from build123d import *

# Parameters (mm, degrees)
F1_DEPTH     = 19.05
F2_T1_DEPTH  = 28.2300180496
F2_T3_DEPTH  = 25.482580603
F2_T5_DEPTH  = 25.9366089247
F2_T7_DEPTH  = 47.5485210799
F2_T9_DEPTH  = 32.7314977927
F2_T11_DEPTH = 59.1455336843
F2_T13_DEPTH = 52.8213628452
F2_T15_DEPTH = 21.9875710363
F2_T17_DEPTH = 46.4468482438
F2_T19_DEPTH = 29.758572197
F3_R         = 5.08
F5_W         = 6.35
F5_H         = 12.7
F6_DEPTH     = 303.0582275594


# Not quite as in the source:
# - a fillet or chamfer that OpenCascade refuses, or shapes differently, is made with other operations: its cross-section is extruded or revolved along the edge and cut away or added


with BuildPart() as f1:
    # F0 (on Front) → F1 (new body)
    with BuildSketch(Plane.XZ):
        Polygon((-45.0859302655, 0.4672128707), (-34.340060316, 0.4672128707), (-31.5367905423, 4.9057230353), (-31.5367905423, 9.1106286272), (-31.5367905423, 12.6147158444), (-29.4343372807, 13.7827442959), (-19.1556811333, 15.8851970918), (-16.2193404098, 14.3601642462), (-11.9138995651, 12.6147158444), (-11.9138995651, 9.1106286272), (-11.9138995651, 7.4753854424), (-9.811447002, 1.5152803213), (-6.0737542808, 0), (0, 0), (0, 2.3983575983), (1.1680293828, 5.2794977153), (1.1680293828, 9.1106286272), (1.1680293828, 12.6147158444), (0, 17.2868324444), (-1.4916199837, 18.4976548306), (3.0368734151, 29.6679423191), (4.9057211727, 31.0695767403), (6.0737496242, 31.770395115), (8.4476916948, 31.5367886797), (9.3986034807, 33.8823718767), (12.8483185545, 32.4838392109), (15.1843773201, 31.5367886797), (18.6884636059, 40.1802044362), (14.483560808, 40.1802044362), (14.483560808, 42.2826576978), (12.8483185545, 42.7498687059), (12.1475020424, 44.1515035927), (8.1762028858, 44.1515035927), (5.3729321808, 44.1515035927), (1.1680293828, 44.1515035927), (1.1680293828, 42.2826576978), (-1.4016367495, 40.4138118029), (-3.9712996222, 38.3113585413), (-14.7171695717, 38.3113585413), (-22.192556411, 38.3113585413), (-28.7335207686, 38.3113585413), (-38.0777539685, 35.5080878362), (-43.684293516, 32.4712125584), (-49.0572275594, 27.7990954928), (-49.0572275594, 14.9507736787), (-49.0572275594, 9.1106286272), align=None)
    extrude(amount=F1_DEPTH)

    # F2: fillet of radius 12.5094889948 on 10 edges, made by hand

    # F2_s2 → F2_t1 (cut)
    with BuildSketch(Plane.XZ.offset(-4.5900090248)):
        with BuildLine():
            ThreePointArc((-30.4920932473, 37.7837866574), (-28.7140598467, 38.1787628389), (-26.8975171587, 38.3113585413))
            Line((-26.8975171587, 38.3113585413), (-28.7335207686, 38.3113585413))
            Line((-28.7335207686, 38.3113585413), (-30.4920932473, 37.7837866574))
        make_face()
    extrude(amount=F2_T1_DEPTH, mode=Mode.SUBTRACT)

    # F2_s4 → F2_t3 (cut)
    with BuildSketch(Plane.XZ.offset(-3.2162903015)):
        with BuildLine():
            ThreePointArc((-39.2089772844, 34.8953419361), (-38.0524286269, 35.4471609705), (-36.8454950389, 35.8777656133))
            Line((-36.8454950389, 35.8777656133), (-38.0777539685, 35.5080878362))
            Line((-38.0777539685, 35.5080878362), (-39.2089772844, 34.8953419361))
        make_face()
    extrude(amount=F2_T3_DEPTH, mode=Mode.SUBTRACT)

    # F2_s6 → F2_t5 (cut)
    with BuildSketch(Plane.XZ.offset(-3.4433044624)):
        with BuildLine():
            ThreePointArc((-42.4732255071, 33.1272076629), (-43.6412308258, 32.4090824128), (-44.7236280922, 31.5674432638))
            Line((-44.7236280922, 31.5674432638), (-43.684293516, 32.4712125584))
            Line((-43.684293516, 32.4712125584), (-42.4732255071, 33.1272076629))
        make_face()
    extrude(amount=F2_T5_DEPTH, mode=Mode.SUBTRACT)

    # F2_s8 → F2_t7 (cut)
    with BuildSketch(Plane.XZ.offset(-14.2492605399)):
        with BuildLine():
            ThreePointArc((-49.0572275594, 22.0993912768), (-47.9313005389, 27.2860888474), (-44.7561994839, 31.5391203114))
            Line((-44.7561994839, 31.5391203114), (-49.0572275594, 27.7990954928))
            Line((-49.0572275594, 27.7990954928), (-49.0572275594, 22.0993912768))
        make_face()
    extrude(amount=F2_T7_DEPTH, mode=Mode.SUBTRACT)

    # F2_s10 → F2_t9 (cut)
    with BuildSketch(Plane.XZ.offset(-6.8407488963)):
        with BuildLine():
            ThreePointArc((-49.0572275594, 11.8469281858), (-48.7682894076, 9.1738303565), (-47.9148224607, 6.6242163797))
            Line((-47.9148224607, 6.6242163797), (-49.0572275594, 9.1106286272))
            Line((-49.0572275594, 9.1106286272), (-49.0572275594, 11.8469281858))
        make_face()
    extrude(amount=F2_T9_DEPTH, mode=Mode.SUBTRACT)

    # F2_s12 → F2_t11 (cut)
    with BuildSketch(Plane.XZ.offset(-20.0477668422)):
        with BuildLine():
            ThreePointArc((-37.0668235286, 0.4672128707), (-43.8178922977, 2.4453018928), (-48.4339074248, 7.7539900595))
            Line((-48.4339074248, 7.7539900595), (-45.0859302655, 0.4672128707))
            Line((-45.0859302655, 0.4672128707), (-37.0668235286, 0.4672128707))
        make_face()
    extrude(amount=F2_T11_DEPTH, mode=Mode.SUBTRACT)

    # F2_s14 → F2_t13 (cut)
    with BuildSketch(Plane.XZ.offset(-16.8856814226)):
        with BuildLine():
            ThreePointArc((-31.5367905423, 4.9057230353), (-35.825391148, 1.6309728064), (-41.0943328851, 0.4672128707))
            Line((-41.0943328851, 0.4672128707), (-34.340060316, 0.4672128707))
            Line((-34.340060316, 0.4672128707), (-31.5367905423, 4.9057230353))
        make_face()
    extrude(amount=F2_T13_DEPTH, mode=Mode.SUBTRACT)

    # F2_s16 → F2_t15 (cut)
    with BuildSketch(Plane.XZ.offset(-1.4687855182)):
        with BuildLine():
            ThreePointArc((-15.6748678973, 14.139432221), (-16.2135660804, 14.3726858024), (-16.7407283206, 14.6309549221))
            Line((-16.7407283206, 14.6309549221), (-16.2193404098, 14.3601642462))
            Line((-16.2193404098, 14.3601642462), (-15.6748678973, 14.139432221))
        make_face()
    extrude(amount=F2_T15_DEPTH, mode=Mode.SUBTRACT)

    # F2_s18 → F2_t17 (cut)
    with BuildSketch(Plane.XZ.offset(-13.6984241219)):
        with BuildLine():
            ThreePointArc((-6.0737542808, 0), (-9.4531651589, 2.8427255588), (-11.6342326331, 6.6825759671))
            Line((-11.6342326331, 6.6825759671), (-9.811447002, 1.5152803213))
            Line((-9.811447002, 1.5152803213), (-6.0737542808, 0))
        make_face()
    extrude(amount=F2_T17_DEPTH, mode=Mode.SUBTRACT)

    # F2_s20 → F2_t19 (cut)
    with BuildSketch(Plane.XZ.offset(-5.3542860985)):
        with BuildLine():
            ThreePointArc((-11.2014295993, 5.4556509826), (-11.7344956192, 7.5061006875), (-11.9138995651, 9.6170998818))
            Line((-11.9138995651, 9.6170998818), (-11.9138995651, 7.4753854424))
            Line((-11.9138995651, 7.4753854424), (-11.2014295993, 5.4556509826))
        make_face()
    extrude(amount=F2_T19_DEPTH, mode=Mode.SUBTRACT)

    # F3
    f3_edges = [f1.edges().sort_by_distance(p)[0] for p in [
        (16.93642, 0, 35.858497),
        (16.93642, -19.05, 35.858497),
    ]]
    fillet(f3_edges, radius=F3_R)

    # F5 (on offset) → F6 (cut, through all)
    with BuildSketch(Plane.YZ.offset(254)):
        with Locations((-9.525, 6.35)):
            Rectangle(F5_W, F5_H)
    extrude(amount=-F6_DEPTH, mode=Mode.SUBTRACT)


solid = f1.part
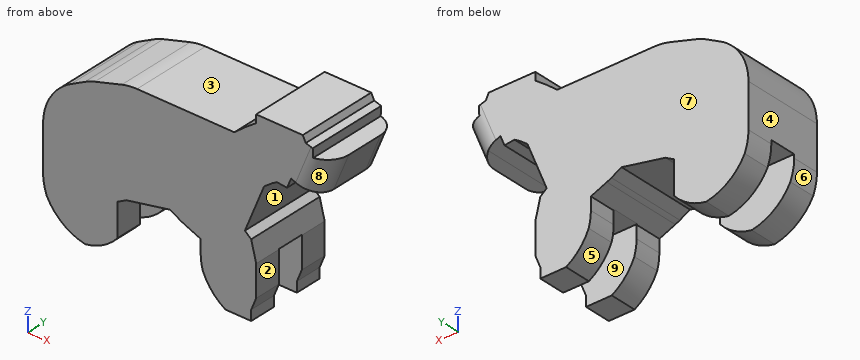
Geometry check sheet. Reference: the model listing, model coordinates, mm. Face numbers are marked on the shaded views. A direction names the side the tool comes from. Round coordinates to 2 decimals unless told otherwise and drop trailing zeros. Loops run counter-clockwise (first coordinate to the right, second up) from the corner with the lowest first, then second, coordinate; pieces in that order, holes last.
Item 1: Cross-section at D-D on z = 20. Record the boundary of the cut face in (x, y), then the cut area to 3 significant figures.
Item 2: Thickness scan on line 1 (X direction, y = -17.75, z = 11.5); line 2 (Y direction, x = -35, z = 6); line 3 (X direction, y = -16, z = 13). Record the ranges inside material, lowest first.
Item 3: Access from +Z, -Z, +X, -X, +Y, -Y to the whole of each face (thin tool, end or side, straight path). Record for the marked faces 1, 2, 3, 4 and 5.
Item 4: Cross-section at A-A on z = 8. Record the boundary of the cut face in (x, y).
Item 5: Mould release check, pull along Y, two halves, no side actions. Record for the marked faces 6, 7, 8 and 9: pulls with the +Y half, pulls with the -Y half, needs draft (parallel to the pull), parting line crosses it, or undercut.
Item 6: Gauge pin test, flat ends, axial feed: pin 1 (1.9 mm diameter, centred on y = -14.5, z = 8, fed in from +X); pin 2 (2 mm diameter, centred on x = 16.5, y = -7, fed in from +Z); pin 3 (0.6 mm diameter, centred on y = -5, z = 41, fed in from +X). Record the tip position at first contact, or that the pin passes through.
Item 7: Cross-section at C-C on x = -33.5. Record the boundary of the cut face in (y, z).
Answer sheet:
1. outline: (-49.06, -19.05) - (-0.88, -19.05) - (-0.88, 0) - (-49.06, 0) - close
1. area: 918 mm2
2. line 1: x = -49.05 to -31.54, -11.91 to 1.17
2. line 2: y = -19.05 to -12.7, -6.35 to 0
2. line 3: x = -49.06 to -30.84, -12.86 to 1.07
3. face 1: +X, +Y, -Y
3. face 2: -Z, +X, +Y, -Y
3. face 3: +Z, -X, +Y, -Y
3. face 4: +Z, -Z, -X, +Y, -Y
3. face 5: -Z, +Y, -Y
4. outline: (-48.45, -19.05) - (-31.54, -19.05) - (-31.54, -12.7) - (-48.45, -12.7) - close; (-48.45, -6.35) - (-31.54, -6.35) - (-31.54, 0) - (-48.45, 0) - close; (-11.81, -19.05) - (1.17, -19.05) - (1.17, -12.7) - (-11.81, -12.7) - close; (-11.81, -6.35) - (1.17, -6.35) - (1.17, 0) - (-11.81, 0) - close
5. face 6: needs draft
5. face 7: pulls with the +Y half
5. face 8: pulls with the -Y half
5. face 9: undercut
6. pin 1: stops at x = 1.17
6. pin 2: stops at z = 40.18
6. pin 3: stops at x = 14.48
7. outline: (-19.05, 3.04) - (-12.7, 3.04) - (-12.7, 12.7) - (-6.35, 12.7) - (-6.35, 3.04) - (0, 3.04) - (0, 36.88) - (-19.05, 36.88) - close
